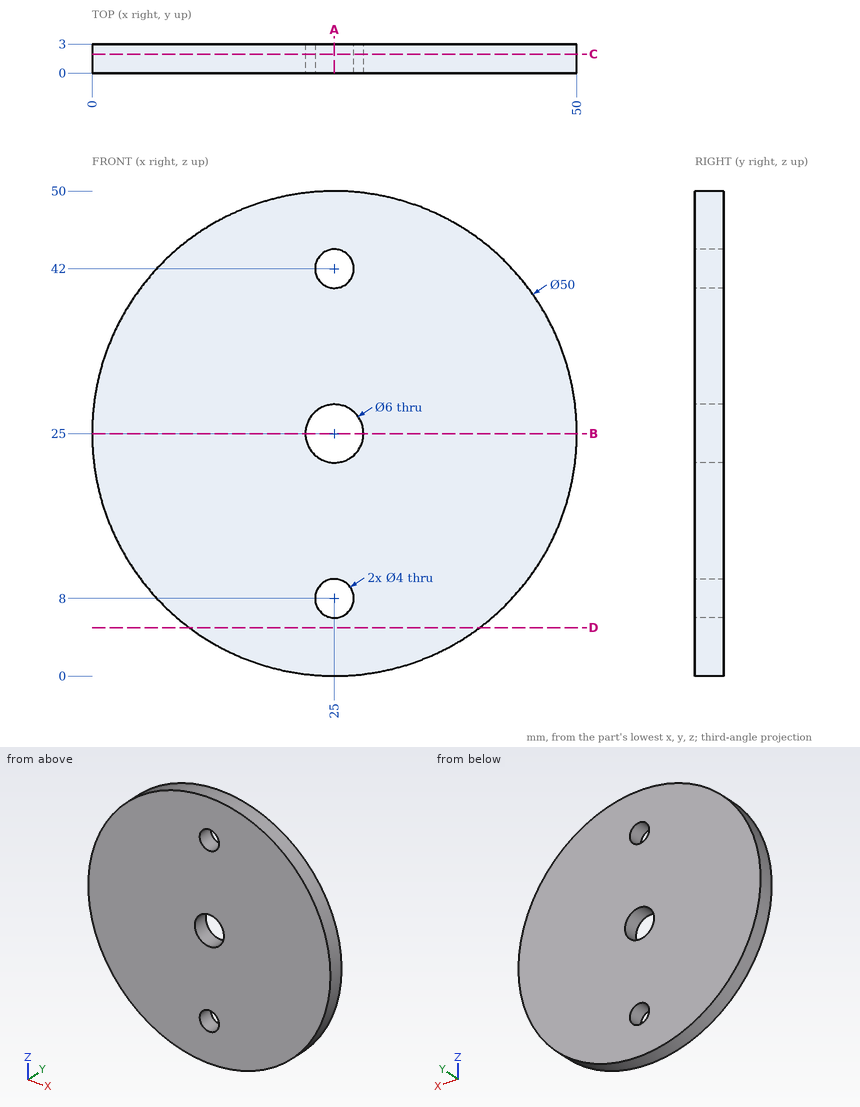
Answer from the drawing. Dimensions are ordinates in mm from the lowest x, y and z of the part. Give positions to 0.01 mm unless a question says otherwise; leave off trailing zeros. Loops run counter-clockwise (first coordinate to the right, second up) from the corner with the lowest first, then second, coordinate; pieces in that order, holes last.
Item 1: The part is cut by section D-D (z = 5). Write down the section's boundary in (x, y), and give its area (3 significant figures).
Item 2: The part is cut by section C-C (y = 1.95). Write down the section's boundary in (x, z), and give its area (3 significant figures).
Item 3: Find the intervals of material crossed by line 1 along Z through (x, y) = (25, 2); line 2 along Z through (x, y) = (24.5, 2.05) (1 decimal); line 3 along Z through (x, y) = (45, 0.3), in increasing order.
Item 4: The part is cut by section A-A (x = 25). Write down the section's boundary in (y, z), and give its area (3 significant figures).
Item 5: The part is cut by section B-B (z = 25). Write down the section's boundary in (x, y).
Item 6: Each of these flat-tipped pins is pushed along its axis until it touches: pin 1 Ø1 at (y, z) = (1, 6.5) entering from -X; pin 2 Ø2.5 at (x, z) = (25, 8) entering from -Y. Where does it stop, or does it pass through?
Taken from the geometry:
1. outline: (10, 0) - (40, 0) - (40, 3) - (10, 3) - close
1. area: 90.0 mm2
2. outline: circle Ø50 at (25, 25); hole circle Ø6 at (25, 25); hole circle Ø4 at (25, 8); hole circle Ø4 at (25, 42)
2. area: 1,910 mm2
3. line 1: z = 0 to 6, 10 to 22, 28 to 40, 44 to 50
3. line 2: z = 0 to 6.1, 9.9 to 22, 28 to 40.1, 43.9 to 50
3. line 3: z = 10 to 40
4. outline: (0, 0) - (3, 0) - (3, 6) - (0, 6) - close; (0, 10) - (3, 10) - (3, 22) - (0, 22) - close; (0, 28) - (3, 28) - (3, 40) - (0, 40) - close; (0, 44) - (3, 44) - (3, 50) - (0, 50) - close
4. area: 108 mm2
5. outline: (0, 0) - (22, 0) - (22, 3) - (0, 3) - close; (28, 0) - (50, 0) - (50, 3) - (28, 3) - close
6. pin 1: stops at x = 7.65
6. pin 2: passes through
